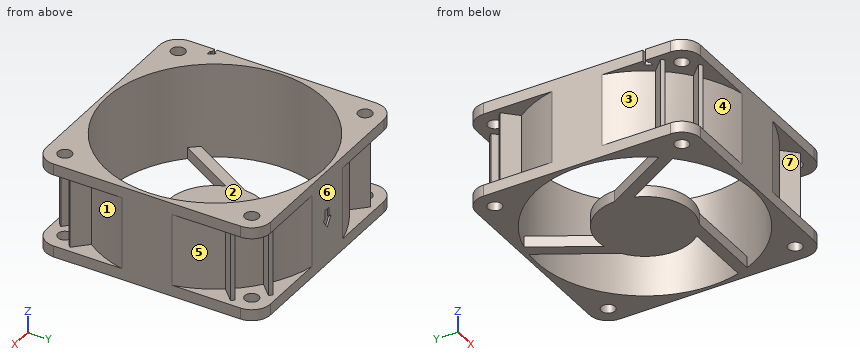
```python
from build123d import *

# Parameters (mm, degrees)
SKETCH_BODY_R                       = 29
BODY_DEPTH                          = 25.4
SKETCH_CUT_BODY_W                   = 19.4
SKETCH_CUT_BODY_H                   = 9.605339059
REINFORCMENT_STRIP_REACH            = 51.449
CIRPATTERN_REINFORCMENT_STRIP_COUNT = 4
SKETCH_FIXING_HOLE_R                = 1.85
FIXING_HOLE_DEPTH                   = 50.44855913
CIRPATTERN_FIXING_HOLE_COUNT        = 4
BONE_DEPTH                          = 3
CIRPATTERN_BONE_COUNT               = 3
CUT_REINFORCMENT_STRIP_HOLE_DEPTH   = 22.4
SKETCH_FIXING_PLATE_FAN_R           = 12.5
FIXING_PLATE_FAN_DEPTH              = 3
AIR_EXHAUST_DEPTH                   = 72.312060691


with BuildPart() as part:
    # Sketch-Body → Body (new body)
    with BuildSketch(Plane.XY):
        with BuildLine():
            Line((-25, -30), (25, -30))
            ThreePointArc((25, -30), (28.535533906, -28.535533906), (30, -25))
            Line((30, -25), (30, 25))
            ThreePointArc((30, 25), (28.535533906, 28.535533906), (25, 30))
            Line((25, 30), (-25, 30))
            ThreePointArc((-25, 30), (-28.535533906, 28.535533906), (-30, 25))
            Line((-30, 25), (-30, -25))
            ThreePointArc((-30, -25), (-28.535533906, -28.535533906), (-25, -30))
        make_face()
        Circle(SKETCH_BODY_R, mode=Mode.SUBTRACT)
    extrude(amount=BODY_DEPTH)

    # Sketch-Cut-Body → Cut-Body (revolve, cut)
    with BuildSketch(Plane(origin=(0, 0, 0), x_dir=(0, 0, -1), z_dir=(1, 0, 0))):
        with Locations((-12.7, 35.55266953)):
            Rectangle(SKETCH_CUT_BODY_W, SKETCH_CUT_BODY_H)
    revolve(axis=Axis((0, 0, 25.4), (0, 0, -1)), mode=Mode.SUBTRACT)

    # Sketch-Reinforcment-Strip → Reinforcment-Strip (add, up to next)
    with BuildSketch(Plane.XY, mode=Mode.PRIVATE) as reinforcment_strip_sk1:
        with BuildLine():
            Line((24.452034569, 17.380966757), (28.535533906, 21.464466094))
            Line((28.535533906, 21.464466094), (27.779609669, 22.220390331))
            Line((27.779609669, 22.220390331), (23.809915661, 18.250696322))
            ThreePointArc((23.809915661, 18.250696322), (24.13489315, 17.818724214), (24.452034569, 17.380966757))
        make_face()
    reinforcment_strip_tool1 = extrude(reinforcment_strip_sk1.sketch, amount=REINFORCMENT_STRIP_REACH, mode=Mode.PRIVATE) - part.part
    # Sketch-Reinforcment-Strip → Reinforcment-Strip (add, up to next)
    with BuildSketch(Plane.XY, mode=Mode.PRIVATE) as reinforcment_strip_sk2:
        with BuildLine():
            Line((17.380966757, 24.452034569), (21.464466094, 28.535533906))
            Line((21.464466094, 28.535533906), (22.220390331, 27.779609669))
            Line((22.220390331, 27.779609669), (18.250696322, 23.809915661))
            ThreePointArc((18.250696322, 23.809915661), (17.818724214, 24.13489315), (17.380966757, 24.452034569))
        make_face()
    reinforcment_strip_tool2 = extrude(reinforcment_strip_sk2.sketch, amount=REINFORCMENT_STRIP_REACH, mode=Mode.PRIVATE) - part.part
    reinforcment_strip_1 = reinforcment_strip_tool1.solids().sort_by_distance((26.147081, 19.828375, 0))[0]
    add(reinforcment_strip_1)
    reinforcment_strip_2 = reinforcment_strip_tool2.solids().sort_by_distance((19.828375, 26.147081, 0))[0]
    add(reinforcment_strip_2)
    reinforcment_strip = reinforcment_strip_1 + reinforcment_strip_2  # Reinforcment-Strip as one shape, for the pattern or mirror that repeats it

    # CirPattern-Reinforcment-Strip: Reinforcment-Strip ×4 about axis
    cirpattern_reinforcment_strip_axis = Axis((0, 0, 0), (0, 0, 1))
    for i in range(1, CIRPATTERN_REINFORCMENT_STRIP_COUNT):
        add(reinforcment_strip.rotate(cirpattern_reinforcment_strip_axis, i * 360 / CIRPATTERN_REINFORCMENT_STRIP_COUNT))

    # Sketch-Fixing-Hole → Fixing-Hole (cut, through all)
    with BuildSketch(Plane.XY):
        with Locations(Location((25, 25, 0), (0, 0, 90))):
            Circle(SKETCH_FIXING_HOLE_R)
    fixing_hole = extrude(amount=FIXING_HOLE_DEPTH, mode=Mode.SUBTRACT)

    # CirPattern-Fixing-Hole: Fixing-Hole ×4 about axis
    cirpattern_fixing_hole_axis = Axis((0, 0, 0), (0, 0, 1))
    for i in range(1, CIRPATTERN_FIXING_HOLE_COUNT):
        add(fixing_hole.rotate(cirpattern_fixing_hole_axis, i * 360 / CIRPATTERN_FIXING_HOLE_COUNT), mode=Mode.SUBTRACT)

    # Sketch-Bone → Bone (add)
    with BuildSketch(Plane.XY):
        with BuildLine():
            Line((-11.764259967, -4.225184898), (-20.920098492, -20.08356241))
            ThreePointArc((-20.920098492, -20.08356241), (-21.989386414, -18.906794681), (-22.992571288, -17.673190589))
            Line((-22.992571288, -17.673190589), (-12.489214378, 0.519157229))
            ThreePointArc((-12.489214378, 0.519157229), (-12.356575173, -1.888133998), (-11.764259967, -4.225184898))
        make_face()
    bone = extrude(amount=BONE_DEPTH)

    # CirPattern-Bone: Bone ×3 about axis
    cirpattern_bone_axis = Axis((0, 0, 0), (0, 0, 1))
    for i in range(1, CIRPATTERN_BONE_COUNT):
        add(bone.rotate(cirpattern_bone_axis, i * 360 / CIRPATTERN_BONE_COUNT))

    # Sketch1 → Cut-Reinforcment-Strip-Hole (cut)
    with BuildSketch(Plane.XY.offset(25.4)):
        with BuildLine():
            Line((-27.430592324, -18.724638365), (-28.841857513, -18.724638365))
            Line((-28.841857513, -18.724638365), (-28.841857513, -18.34833506))
            Line((-28.841857513, -18.34833506), (-30, -18.34833506))
            Line((-30, -18.34833506), (-30, -17.59572845))
            Line((-30, -17.59572845), (-28.841857513, -17.59572845))
            Line((-28.841857513, -17.59572845), (-28.841857513, -17.219425145))
            Line((-28.841857513, -17.219425145), (-28.399663287, -17.219425145))
            ThreePointArc((-28.399663287, -17.219425145), (-27.925271299, -17.978562235), (-27.430592324, -18.724638365))
        make_face()
    extrude(amount=-CUT_REINFORCMENT_STRIP_HOLE_DEPTH, mode=Mode.SUBTRACT)

    # Sketch-Fixing-Plate-Fan → Fixing-Plate-Fan (add)
    with BuildSketch(Plane.XY):
        Circle(SKETCH_FIXING_PLATE_FAN_R)
    extrude(amount=FIXING_PLATE_FAN_DEPTH)

    # Sketch4 → Air-Exhaust (cut, through all)
    with BuildSketch(Plane(origin=(0, 29.5, 0), x_dir=(-1, 0, 0), z_dir=(0, 1, 0))):
        Polygon((0.881634904, 15), (-0.881634904, 15), (-0.881634904, 12.5), (-1.750518846, 12.5), (0, 10), (1.750518846, 12.5), (0.881634904, 12.5), align=None)
    extrude(amount=AIR_EXHAUST_DEPTH, mode=Mode.SUBTRACT)


solid = part.part
```
Work out the finished part from the listing and answer in its coordinate system (mm). Face numbers are marked on the shaded views. A direction names the side the tool comes from. Coordinates: 2 decimals unless noted, no trailing zeros. Write each loop counter-clockwise with the first axis right and the second up, starting at its lowest first coordinate (ties: lowest second). Pieces come first, ordered by that corner, then holes.
Q1. A cutting plane is placed at B-B, the plane y = -16. Give the vertices of the cut face in (x, z).
Q2. Which of the six approach directions +Z, -Z, +X, -X, +Y, -Y give full straight-line access (tool end or side, diameter ignored) to the marked faces 1, 2, 3 and 4?
Q3. A cutting plane is placed at C-C, the plane y = -6. Give the vertices of the cut face in (x, z).
Q4. A cutting plane is placed at A-A, the plane x = -15.5. Give the vertices of the cut face in (y, z), then the cut area to 3 significant figures.
Q5. A cutting plane is placed at D-D, the plane y = 5.5. Give the vertices of the cut face in (x, z).
Q6. Each of these flat-tipped pins is pushed along its axis until it touches: pin 1 Ø12 at (x, y) = (-4.5, -8.5) entering from +Z; pin 2 Ø2 at (x, y) = (-6, 22.5) entering from +Z; pin 3 Ø1 at (y, z) = (-18, 19) entering from +X; pin 4 Ø1.1 at (x, z) = (-28.5, 23.5) entering from +Y. Where does it stop, or does it pass through?
Q7. Find the intervals of material crossed by line 1 (Y direction, x = 25, z = 1.8); line 2 (Z direction, x = -15, y = 27.5); line 3 (X direction, y = -19, z = 21.5), in increasing order.
Q8. Determine the mould class of the marked faces 5, 6 and 7 for opening direction X: released by +X, released by -X, zero draft, split by the parting line, or undercut.
Findings below:
1. outline: (-30, 0) - (-24.19, 0) - (-24.19, 25.4) - (-30, 25.4) - (-30, 22.4) - (-26.26, 22.4) - (-26.26, 3) - (-30, 3) - close; (-22.03, 0) - (-18.56, 0) - (-18.56, 3) - (-22.03, 3) - close; (24.19, 0) - (30, 0) - (30, 3) - (26.26, 3) - (26.26, 22.4) - (30, 22.4) - (30, 25.4) - (24.19, 25.4) - close
2. face 1: +X
2. face 2: +Z
2. face 3: -X
2. face 4: -Y
3. outline: (-30, 0) - (-28.37, 0) - (-28.37, 25.4) - (-30, 25.4) - close; (-16.25, 0) - (-12.79, 0) - (-12.79, 3) - (-16.25, 3) - close; (-10.97, 0) - (10.97, 0) - (10.97, 3) - (-10.97, 3) - close; (28.37, 0) - (30, 0) - (30, 25.4) - (28.37, 25.4) - close
4. outline: (-30, 0) - (-24.51, 0) - (-24.51, 25.4) - (-30, 25.4) - (-30, 22.4) - (-26.56, 22.4) - (-26.56, 3) - (-30, 3) - close; (-10.7, 0) - (-4.7, 0) - (-4.7, 3) - (-10.7, 3) - close; (24.51, 0) - (30, 0) - (30, 3) - (26.56, 3) - (26.56, 22.4) - (30, 22.4) - (30, 25.4) - (24.51, 25.4) - close
4. area: 163 mm2
5. outline: (-30, 0) - (-28.47, 0) - (-28.47, 25.4) - (-30, 25.4) - close; (-11.22, 0) - (11.22, 0) - (11.22, 3) - (-11.22, 3) - close; (28.47, 0) - (30, 0) - (30, 25.4) - (28.47, 25.4) - close
6. pin 1: stops at z = 3
6. pin 2: passes through
6. pin 3: stops at x = 25.57
6. pin 4: stops at y = 29.04
7. line 1: y = -30 to -26.85, -23.15 to -14.7, -11.08 to -8.08, 14.7 to 23.15, 26.85 to 30
7. line 2: z = 0 to 3, 22.4 to 25.4
7. line 3: x = -26.07 to -24.56, -24.18 to -21.91, 21.91 to 24.18, 24.56 to 26.07
8. face 5: released by +X
8. face 6: zero draft
8. face 7: undercut
